Model file for the job. Use its own axes, mm. Face numbers are marked on the shaded views. A direction names the side the tool comes from. Round coordinates to 2 decimals unless told otherwise and drop trailing zeros. Order: outer loops, then holes, each group sorted by start corner. A loop starts at its lowest first (then second) coordinate and runs counter-clockwise, first axis right, second up. Notation, with made-up numbers: M 73.5,-37 L 87.5,-37 A25 ccw 87.5,-2 Z; hole C 44.25,80 d4. An arc over 180 degrees is marked long. Return JSON: item names as keys, results as strings. Group by question number.
Item 1: Probe line 1 along X through (y, z) = (0.3, 18); line 2 along Z through (x, y) = (-4.5, 27.75). List the from-to ranges inside material, lowest first.
Item 2: Slice it at C-C on x = 0.5. Give the number of separate pieces and of enclosed holes in the cut face, then the cut area to 3 significant figures.
Item 3: Pin check, flat tips, straight feed: pin 1 Ø10 at (x, z) = (-0.5, 20.5) entering from +Y; pin 2 Ø5 at (x, y) = (-6.5, 6.5) entering from +Z; pin 3 Ø3.5 at (x, z) = (0, 18) entering from +Y; pin 4 Ø3 at (x, y) = (-4, 11.5) entering from +Z. Stop position of each tip, or through.
Item 4: Slice it at D-D on z = 2.25. Write the cut outline in (x, y), then the cut area to 3 significant figures.
Item 5: Which spindle directions (+Z, -Z, +X, -X, +Y, -Y) get a long thin tool onto all of the face, cutting with end or side? Do the marked faces 1 and 2. Say none if no direction does.
Item 6: Pull direction Z, two halves, no side cores. Call the marked faces 3, 4, 5 and 6: pulls with the +Z half, pulls with the -Z half, needs draft (parallel to the pull), parting line crosses it, or undercut.
Item 7: Slice it at A-A on y = 18. Write the cut outline in (x, z).
Autodesk Inventor part; units mm, degrees
ref_plane "YZ Plane" through (0, 0, 0) normal (1, 0, 0) x (0, 1, 0)
ref_plane "XZ Plane" through (0, 0, 0) normal (0, 1, 0) x (-1, 0, 0)
ref_plane "XY Plane" through (0, 0, 0) normal (0, 0, 1) x (1, 0, 0)
sketch "Эскиз1" plane through (0, 0, 0) normal (0, 0, 1) x (1, 0, 0)
  line L0 (-10, 0) -> (10, 0)
  line L1 (10, 0) -> (10, 20)
  line L2 (0, 30) -> (0, 30)
  line L3 (-10, 20) -> (-10, 0)
  arc A0 (0, 30) -> (-10, 20) centre (0, 20) ccw
  arc A1 (10, 20) -> (0, 30) centre (0, 20) ccw
  line L4 (0, -6.4142) -> (0, 38.4853)
  point P0 (0, 0)
  point P1 (0, 30)
  dimension "d0" = 20
  dimension "d1" = 10
  dimension "d2" = 20
extrude "Пластина1" add sketch "Эскиз1" along normal blind 3
sketch "Эскиз2" plane through (10, 3, 0) normal (0, -1, 0) x (1, 0, 0)
  line L0 (-20, 0) -> (0, 0)
  line L1 (0, 0) -> (0, 30)
  line L2 (0, 30) -> (-20, 30)
  line L3 (-20, 30) -> (-20, 0)
edge flange "Фланец1" height 30 angle 90 thickness 3 bend radius 3 thickness toward (0, -1, 0) relief tear relief width 3 relief depth 1.5 edges at (0, 0, 3) wall of the first edge with corners at (-10, 3, 0) (10, 3, 0) (10, 3, 30) (-10, 3, 30)
bend "Сгиб1"
corner "УглСтык1"
fillet "Сопряжение1" radius 10 2 edges at (-10, 1.5, 30) (10, 1.5, 30)
sketch "Эскиз3" plane through (0, 0, 3) normal (0, 0, 1) x (1, 0, 0)
  line L0 (0, -6) -> (0, 36)
  arc A0 (10, 20) -> (-10, 20) centre (0, 20) ccw
  point P0 (0, 0)
  point P1 (0, 18)
  point P2 (0, 30)
  dimension "d29" = 12
hole "Отверстие1" at (0, 18, 3) direction (0, 0, -1) diameter 5.5 end through all countersink diameter 10.5 countersink angle 90
sketch "Эскиз4" plane through (-10, 3, 6) normal (0, 1, 0) x (1, 0, 0)
  line L0 (0, 0) -> (0, -14)
  arc A0 (0, -14) -> (20, -14) centre (10, -14) ccw
  point P0 (10, 6)
  point P1 (10, -12)
  point P2 (10, -24)
  dimension "d30" = 10
  dimension "d31" = 12
hole "Отверстие2" at (0, 3, 18) direction (0, -1, 0) diameter 5.5 end through all countersink diameter 10.5 countersink angle 90
equation "\"d20\" = Толщина"
equation "\"d3\" = Толщина"
equation "\"d4\" = Ширина_просечки"
equation "\"d5\" = Глубина_просечки"
equation "\"d6\" = Мин_остаток"
equation "\"d7\" = Радиус_перехода"
equation "\"d10\" = Радиус_гибки"
equation "\"d11\" = Размер_просечки"
equation "\"d12\" = Размер_зазора"
equation "\"d13\" = Радиус_Якоби"
equation "\"Радиус_гибки\" = Толщина"
equation "\"Ширина_просечки\" = Толщина"
equation "\"Глубина_просечки\" = 0.5 * Толщина"
equation "\"Размер_просечки\" = 4 * Толщина"
equation "\"Мин_остаток\" = 2 * Толщина"
equation "\"Радиус_перехода\" = Радиус_гибки"
equation "\"Радиус_Якоби\" = Радиус_гибки"
equation "\"Размер_зазора\" = Толщина"
properties part number "скоба"
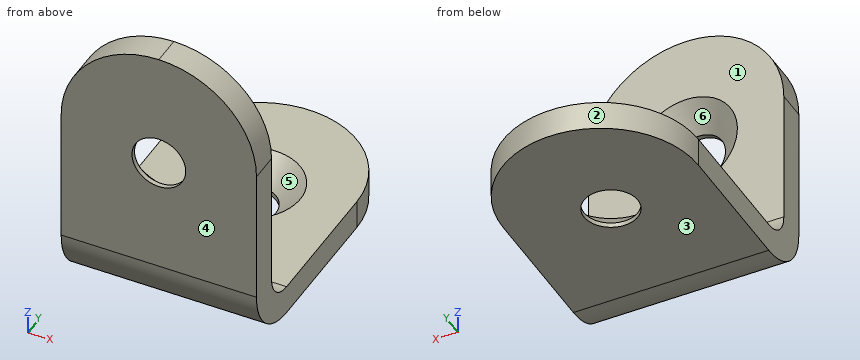
Output values:
{
 "1": {"line 1": "-10 to -2.75, 2.75 to 10", "line 2": "0 to 3"},
 "2": {"separate pieces": "3", "enclosed holes": "0", "area": "120 mm²"},
 "3": {"pin 1": "y = 3", "pin 2": "z = 3.76", "pin 3": "through", "pin 4": "z = 3"},
 "4": {"outline": "M -10,1.32 L 10,1.32 L 10,20 A10 ccw -10,20 Z; hole C 0,18 d9", "area": "467 mm²"},
 "5": {"face 1": "+Z, +X, -X, +Y", "face 2": "+Z, -Z, +Y"},
 "6": {"face 3": "pulls with the -Z half", "face 4": "needs draft", "face 5": "pulls with the +Z half", "face 6": "undercut"},
 "7": {"outline": "M -10,0 L -2.75,0 L -2.75,0.5 L -5.25,3 L -10,3 Z; M 2.75,0 L 10,0 L 10,3 L 5.25,3 L 2.75,0.5 Z"}
}
